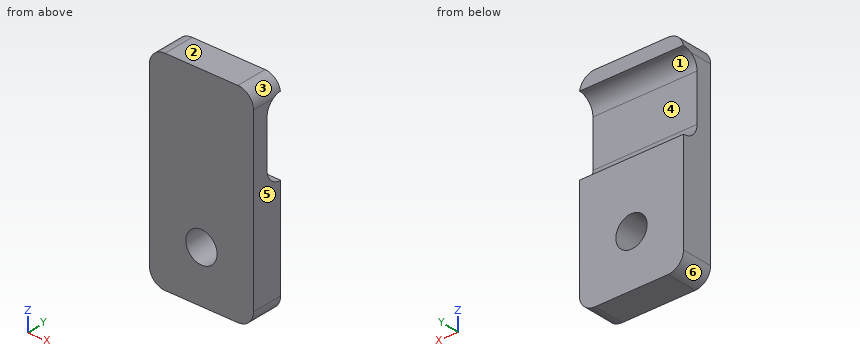
Autodesk Inventor part; units mm, degrees
ref_plane "YZ Plane" through (0, 0, 0) normal (1, 0, 0) x (0, 1, 0)
ref_plane "XZ Plane" through (0, 0, 0) normal (0, 1, 0) x (-1, 0, 0)
ref_plane "XY Plane" through (0, 0, 0) normal (0, 0, 1) x (1, 0, 0)
sketch "Sketch1" plane through (0, 0, 0) normal (0, 1, 0) x (-1, 0, 0)
  line L0 (0, 0) -> (20, 0)
  line L1 (20, 0) -> (20, -40)
  line L2 (20, -40) -> (0, -40)
  line L3 (0, -40) -> (0, 0)
  circle A0 centre (10, -30) radius 3
  dimension "d0" = 20
  dimension "d1" = 40
  dimension "d2" = 6
  dimension "d3" = 10
  dimension "d4" = 10
extrude "Extrusion1" add sketch "Sketch1" along normal blind 6
sketch "Sketch2" plane through (0, 6, 0) normal (0, 1, 0) x (1, 0, 0)
  line L0 (-20, 0) -> (0, 0)
  line L1 (-10, 0) -> (-10, 10)
  line L2 (0, 17.5) -> (-20, 17.5)
  line L3 (-20, 17.5) -> (-20, 2.5)
  line L4 (-20, 2.5) -> (0, 2.5)
  line L5 (0, 2.5) -> (0, 17.5)
  line L6 (0, 17.5) -> (-20, 2.5) construction
  line L7 (-20, 17.5) -> (0, 2.5) construction
  dimension "d7" = 10
  dimension "d8" = 20
  dimension "d9" = 15
extrude "Extrusion2" cut sketch "Sketch2" against normal blind 3
fillet "Fillet1" radius 3 2 edges at (-10, 3, -17.5) (-10, 3, -2.5)
fillet "Fillet2" radius 3 4 edges at (-20, 3, -40) (0, 3, -40) (-20, 3, 0) (0, 3, 0)
properties part number "CableTieDown"
Source: CAD feature listing. Evaluate the final solid. Frame: model axes, mm. Face numbers are marked on the shaded views. A direction names the side the tool comes from. Round coordinates to 2 decimals unless told otherwise and drop trailing zeros. Write each loop counter-clockwise with the first axis right and the second up, starting at its lowest first coordinate (ties: lowest second). Pieces come first, ordered by that corner, then holes. Notation, with made-up numbers: M 67.5,74 L 84.5,74 A31 ccw 84.5,113 Z; hole C 54.5,-2 d9. An arc over 180 degrees is marked long. Use CSV: the item, a comma, the result in double quotes. Start each with the question number.
Q1. First-contact query: P1, Ø5.5, axis at x = -10, z = -30, coming from the -Y side; P2, Ø1.5, axis at x = -5.5, z = -13, coming from the +Y side. Flat tips, straight axial feed; report the tip coordinate or a pass-through.
Q2. Cut plane C-C on y = 2.25. Output: boundary loops of the cut face in (x, z).
Q3. Pull-direction query (Z, two-part tool) for the marked faces 3, 4, 5 and 6; classes: +Z half, -Z half, draft (parallel to the pull), parting line (faces both ways), or undercut.
Q4. Line query: line 1 (Z direction, x = -10, y = 1.8); line 2 (Z direction, x = -10, y = 4.45); line 3 (Z direction, x = -9.25, y = 5.5). Output: solid intervals per line, ascending. Write a range as from..to.
Q5. Access query for the marked faces 1 and 2. Directions: +Z, -Z, +X, -X, +Y, -Y. A direction counts if a zero-diameter tool reaches every point of the face in a straight line with its end or side. Return the directions, or none.
Q6. Cut plane A-A on z = -30. Output: boundary loops of the cut face in (x, y).
Results found:
1,P1,"through"
1,P2,"y = 3"
2,outline,"M -20,-37 A3 ccw -17,-40 L -3,-40 A3 ccw 0,-37 L 0,-3 A3 ccw -3,0 L -17,0 A3 ccw -20,-3 Z; hole C -10,-30 d6"
3,face 3,"+Z half"
3,face 4,"undercut"
3,face 5,"draft"
3,face 6,"-Z half"
4,line 1,"-40..-33, -27..0"
4,line 2,"-40..-33, -27..-17.07, -2.93..0"
4,line 3,"-40..-32.9, -27.1..-17.46, -2.54..0"
5,face 1,"+X, -X, +Y"
5,face 2,"+Z, +X, -X, +Y, -Y"
6,outline,"M -20,0 L -13,0 L -13,6 L -20,6 Z; M -7,0 L 0,0 L 0,6 L -7,6 Z"
